Here's how the part is built. I have some questions about the finished solid (model axes, mm). Give positions to 0.01 mm unless a question says otherwise; leave off trailing zeros. Loops run counter-clockwise (first coordinate to the right, second up) from the corner with the lowest first, then second, coordinate; pieces in that order, holes last. Notation, with made-up numbers: (-33, -11) - (-15, -11) arc R10 cw to (-15, 5) - close; hole circle Ø9 at (39, -16.5). An arc over 180 degrees is marked (long way). Put each result on its own line as item: value. Start each with the question number.
from build123d import *

# Parameters (mm, degrees)
BOSS_EXTRU_1_START      = -50
ESQUISSE1_R             = 60
BOSS_EXTRU_1_DEPTH      = 80
COQUE1_T                = -5
BOSS_EXTRU_2_START      = 15
ESQUISSE2_R             = 60
BOSS_EXTRU_2_DEPTH      = 15
ESQUISSE3_R             = 17.5
ENL_V_MAT_EXTRU_1_DEPTH = 20
ESQUISSE4_R             = 20
ENL_V_MAT_EXTRU_2_DEPTH = 1
CONG_1_R                = 10
CONG_2_R                = 10
ECHELLE1_SCALE          = 0.25


with BuildPart() as part:
    # Esquisse1 → Boss.-Extru.1 (new body)
    with BuildSketch(Plane.XY.offset(BOSS_EXTRU_1_START)):
        Circle(ESQUISSE1_R)
    extrude(amount=BOSS_EXTRU_1_DEPTH)

    # Coque1
    coque1_openings = [part.faces().sort_by_distance(p)[0] for p in [
        (0, 0, 30),
    ]]
    offset(amount=COQUE1_T, openings=coque1_openings, kind=Kind.INTERSECTION)

    # Esquisse2 → Boss.-Extru.2 (add)
    with BuildSketch(Plane(origin=(0, 0, -50), x_dir=(-1, 0, 0), z_dir=(0, 0, -1)).offset(BOSS_EXTRU_2_START)):
        Circle(ESQUISSE2_R)
    extrude(amount=-BOSS_EXTRU_2_DEPTH)

    # Esquisse3 → Enlèv. mat.-Extru.1 (cut)
    with BuildSketch(Plane(origin=(0, 0, -65), x_dir=(-1, 0, 0), z_dir=(0, 0, -1))):
        Circle(ESQUISSE3_R)
    extrude(amount=-ENL_V_MAT_EXTRU_1_DEPTH, mode=Mode.SUBTRACT)

    # Esquisse4 → Enlèv. mat.-Extru.2 (cut)
    with BuildSketch(Plane.XY.offset(-45)):
        Circle(ESQUISSE4_R)
    extrude(amount=-ENL_V_MAT_EXTRU_2_DEPTH, mode=Mode.SUBTRACT)

    # Congé1
    cong_1_edges = [part.edges().sort_by_distance(p)[0] for p in [
        (60, 0, -65),
    ]]
    fillet(cong_1_edges, radius=CONG_1_R)

    # Congé2
    # the kernel refuses this fillet: 10 mm, written as the material it takes off along each edge
    with BuildSketch(Plane(origin=(0, 0, 30), x_dir=(1, 0, 0), z_dir=(0, -1, 0))) as cong_2_piece_1:
        with BuildLine():
            CenterArc((50, -8.660254038), CONG_2_R, 0, 60)
            Line((55, 0), (55.1, 0.173205081))
            ThreePointArc((55.1, 0.173205081), (57.5, 0.2), (60, 0.2))
            Line((60, 0.2), (60.2, 0))
            Line((60.2, 0), (60.2, -8.660254038))
            Line((60.2, -8.660254038), (60, -8.660254038))
        make_face()
    revolve(axis=Axis((0, 0, 30), (0, 0, 1)), mode=Mode.SUBTRACT)


with BuildPart() as part_1:
    # Echelle1: scaled about (0, 0, -36.474067002)
    add(part.part.scale(ECHELLE1_SCALE).moved(Location((0, 0, -27.355550251))))


solid = part_1.part
1) I need wall thicknesses on line 1 (X direction, y = 0, z = -26); line 2 (Y direction, x = 0, z = -38.7). Which ranges of each line are inside material? Lowest first, please.
2) I'm going to push flat-ended pins straight in: P1, Ø10, axis at x = -1.5, z = -32.5, coming from the -Y side; P2, Ø12, axis at x = 11, z = -38, coming from the +Y side; P3, Ø6, axis at y = -5, z = -40.5, coming from the -X side; P4, Ø6, axis at x = 0, y = 0, coming from the +Z side. Where does each tip first touch, or does it pass through?
3) Suppose I cut it at A-A on x = 0. Please give me the cut outline in (y, z) (3 decimals).
4) Suppose I cut it at D-D on z = -42. Please give me the cut outline in (x, y) (3 decimals), plus the area to 3 significant figures.
5) Suppose I cut it at C-C on z = -27.75. Please give me the cut outline in (x, y), plus the area to 3 significant figures.
6) Thinking about a two-plate mould opening in X: for faces 1 (the flat face through (0, -5, -43.606)), 2 (the cylindrical face through (3.472, -2.662, -41.264)), which applies, pulls with the +X half, pulls with the -X half, needs draft (parallel to the pull), parting line crosses it, or undercut?
Ans:
1. line 1: x = -15 to -13.75, 13.75 to 15
1. line 2: y = -15 to -5, 5 to 15
2. P1: stops at y = -15
2. P2: stops at y = 14.14
2. P3: stops at x = -14.87
2. P4: passes through
3. outline: (-15, -41.106) arc R2.5 ccw to (-12.5, -43.606) - (-4.375, -43.606) - (-4.375, -38.856) - (-5, -38.856) - (-5, -38.606) - (-13.75, -38.606) - (-13.75, -19.856) arc R2.5 ccw to (-15, -22.021) - close; (4.375, -43.606) - (12.5, -43.606) arc R2.5 ccw to (15, -41.106) - (15, -22.021) arc R2.5 ccw to (13.75, -19.856) - (13.75, -38.606) - (5, -38.606) - (5, -38.856) - (4.375, -38.856) - close
4. outline: circle Ø29.669 at (0, 0); hole circle Ø8.75 at (0, 0)
4. area: 631 mm²
5. outline: circle Ø30 at (0, 0); hole circle Ø27.5 at (0, 0)
5. area: 113 mm²
6. face 1: needs draft
6. face 2: undercut
